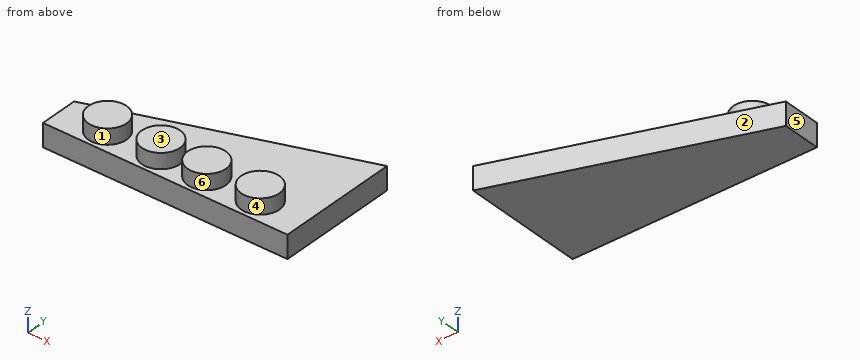
from build123d import *

# Parameters (mm, degrees)
F1_DEPTH = 3
F3_DEPTH = 2
F4_DEPTH = 2


# Not quite as in the source:
# - a feature names something its author has since deleted; it is built from what else it names


with BuildPart() as f1:
    # F0 (on Top) → F1 (new body)
    with BuildSketch(Plane.XY):
        Polygon((-16, -8), (16, -8), (16, 8), (-16, -3), align=None)
    extrude(amount=F1_DEPTH)

    # F2 (on face) → F3 (join)
    with BuildSketch(Plane.XY.offset(3)):
        with BuildLine():
            Line((7.5, -5), (12.5, -5))
            ThreePointArc((12.5, -5), (10, -2.5), (7.5, -5))
        make_face()
        with BuildLine():
            ThreePointArc((7.5, -5), (10, -7.5), (12.5, -5))
            Line((12.5, -5), (7.5, -5))
        make_face()
        with BuildLine():
            ThreePointArc((-7.5, -5), (-10, -2.5), (-12.5, -5))
            Line((-12.5, -5), (-7.5, -5))
        make_face()
        with BuildLine():
            Line((-7.5, -5), (-12.5, -5))
            ThreePointArc((-12.5, -5), (-10, -7.5), (-7.5, -5))
        make_face()
    extrude(amount=F3_DEPTH)

    # F2 (on face) → F4 (join)
    with BuildSketch(Plane.XY.offset(3)):
        with BuildLine():
            Line((7.5, -5), (12.5, -5))
            ThreePointArc((12.5, -5), (10, -2.5), (7.5, -5))
        make_face()
        with BuildLine():
            ThreePointArc((-12.5, -5), (-10, -7.5), (-7.5, -5))
            Line((-7.5, -5), (-12.5, -5))
        make_face()
        with BuildLine():
            Line((-12.5, -5), (-7.5, -5))
            ThreePointArc((-7.5, -5), (-10, -2.5), (-12.5, -5))
        make_face()
        with BuildLine():
            ThreePointArc((-5.5, -5), (-3, -7.5), (-0.5, -5))
            Line((-0.5, -5), (-5.5, -5))
        make_face()
        with BuildLine():
            Line((-5.5, -5), (-0.5, -5))
            ThreePointArc((-0.5, -5), (-3, -2.5), (-5.5, -5))
        make_face()
        with BuildLine():
            ThreePointArc((0.5, -5), (3, -7.5), (5.5, -5))
            Line((5.5, -5), (0.5, -5))
        make_face()
        with BuildLine():
            Line((0.5, -5), (5.5, -5))
            ThreePointArc((5.5, -5), (3, -2.5), (0.5, -5))
        make_face()
        with BuildLine():
            ThreePointArc((7.5, -5), (10, -7.5), (12.5, -5))
            Line((12.5, -5), (7.5, -5))
        make_face()
    extrude(amount=F4_DEPTH)


solid = f1.part
The listing builds one solid part. Answer for the finished solid, in the listing's coordinates (mm). Face numbers are marked on the shaded views. A direction names the side the tool comes from. Coordinates: 2 decimals unless noted, no trailing zeros. Order: outer loops, then holes, each group sorted by start corner. A loop starts at its lowest first (then second) coordinate and runs counter-clockwise, first axis right, second up.
Q1. Given P1, Ø2, axis at x = -3.5, y = 2, coming from the +Z side; P2, Ø3, axis at x = -2.5, z = 1, coming from the +Y side, each flat-ended and moving along its own axis, determine where each tip first touches the part or whether it passes through.
Q2. A cutting plane is placed at C-C, the plane x = -3. Write down the section's boundary in (y, z).
Q3. A cutting plane is placed at D-D, the plane x = 11. Write down the section's boundary in (y, z).
Q4. For a pull along X with two mould halves and no side action, classify the marked faces 3, 4, 5 and 6 as pulls with the +X half, pulls with the -X half, needs draft (parallel to the pull), parting line crosses it, or undercut.
Q5. Which of the six approach directions +Z, -Z, +X, -X, +Y, -Y give full straight-line access (tool end or side, diameter ignored) to the marked faces 1 and 2?
Q6. A cutting plane is placed at A-A, the plane y = -5. Write down the section's boundary in (x, z).
Q7. A cutting plane is placed at B-B, the plane z = 3.3. Write down the section's boundary in (x, y).
Q8. Consider line 1 (X direction, y = -7.25, z = 4.2); line 2 (Z direction, x = 8, y = 4.25); line 3 (Y direction, x = -10, z = 3.85). Determine where each line is inside the solid, lowest interval first.
Answers follow:
1. P1: stops at z = 3
1. P2: stops at y = 2.16
2. outline: (-8, 0) - (1.47, 0) - (1.47, 3) - (-2.5, 3) - (-2.5, 5) - (-7.5, 5) - (-7.5, 3) - (-8, 3) - close
3. outline: (-8, 0) - (6.28, 0) - (6.28, 3) - (-2.71, 3) - (-2.71, 5) - (-7.29, 5) - (-7.29, 3) - (-8, 3) - close
4. face 3: needs draft
4. face 4: undercut
4. face 5: pulls with the -X half
4. face 6: undercut
5. face 1: +Z
5. face 2: +Z, -Z, -X, +Y
6. outline: (-16, 0) - (16, 0) - (16, 3) - (12.5, 3) - (12.5, 5) - (7.5, 5) - (7.5, 3) - (5.5, 3) - (5.5, 5) - (0.5, 5) - (0.5, 3) - (-0.5, 3) - (-0.5, 5) - (-5.5, 5) - (-5.5, 3) - (-7.5, 3) - (-7.5, 5) - (-12.5, 5) - (-12.5, 3) - (-16, 3) - close
7. outline: circle Ø5 at (-10, -5); circle Ø5 at (-3, -5); circle Ø5 at (3, -5); circle Ø5 at (10, -5)
8. line 1: x = -11.09 to -8.91, -4.09 to -1.91, 1.91 to 4.09, 8.91 to 11.09
8. line 2: z = 0 to 3
8. line 3: y = -7.5 to -2.5
